Work out the finished part from the listing and answer in its coordinate system (mm). Round coordinates to 2 decimals unless told otherwise and drop trailing zeros. Loops run counter-clockwise (first coordinate to the right, second up) from the corner with the lowest first, then second, coordinate; pieces in that order, holes last.
from build123d import *

# Parameters (mm, degrees)
F0_W       = 106.68
F0_H       = 208.28
F1_DEPTH   = 2.54
F2_SIZE    = 52.07
F3_SIZE2   = 52.2153074575
F3_SIZE    = 101.6
F3_2_SIZE2 = 52.2153074575
F3_2_SIZE  = 101.6


with BuildPart() as f1:
    # F0 (on Top) → F1 (new body)
    with BuildSketch(Plane.XY):
        Rectangle(F0_W, F0_H)
    extrude(amount=F1_DEPTH)

    # F2
    f2_edges = [f1.edges().sort_by_distance(p)[0] for p in [
        (-53.34, -104.14, 1.27),
        (53.34, -104.14, 1.27),
    ]]
    chamfer(f2_edges, length=F2_SIZE)

    # F3
    f3_edges = [f1.edges().sort_by_distance(p)[0] for p in [
        (-53.34, 104.14, 1.27),
    ]]
    f3_side = f1.faces().sort_by_distance((-53.34, 26.035, 1.27))[0]
    chamfer(f3_edges, length=F3_SIZE, length2=F3_SIZE2, reference=f3_side)

    # F3#2
    f3_2_edges = [f1.edges().sort_by_distance(p)[0] for p in [
        (53.34, 104.14, 1.27),
    ]]
    f3_2_side = f1.faces().sort_by_distance((53.34, 26.035, 1.27))[0]
    chamfer(f3_2_edges, length=F3_2_SIZE, length2=F3_2_SIZE2, reference=f3_2_side)


solid = f1.part
Item 1: Section A-A, the plane z = 1.3 is taken. Give the vertices of the cut face in (x, y), plus the area to 3 significant figures.
Item 2: Section C-C, the plane x = -6 is taken. Give the vertices of the cut face in (y, z).
Item 3: Section B-B, the plane y = -67.5 is taken. Give the vertices of the cut face in (x, z), plus the area to 3 significant figures.
Item 4: Straight lines are drawn through the part: line 1 (Y direction, x = 7, z = 1.55); line 2 (X direction, y = -63, z = 0.35); line 3 (X direction, y = 87, z = 1.25). For each, find the intervals that lie inside material, in ascending order.
Item 5: Each of these flat-tipped pins is pushed along its axis until it touches: P1, Ø1, axis at y = 33, z = 2, coming from the +X side; P2, Ø1.5, axis at y = 77, z = 0.5, coming from the -X side. Where does it stop, or does it pass through?
Answer below:
1. outline: (-53.34, -52.07) - (-1.27, -104.14) - (1.27, -104.14) - (53.34, -52.07) - (53.34, 2.54) - (1.12, 104.14) - (-1.12, 104.14) - (-53.34, 2.54) - close
1. area: 14,200 mm2
2. outline: (-99.41, 0) - (94.65, 0) - (94.65, 2.54) - (-99.41, 2.54) - close
3. outline: (-37.91, 0) - (37.91, 0) - (37.91, 2.54) - (-37.91, 2.54) - close
3. area: 193 mm2
4. line 1: y = -98.41 to 92.71
4. line 2: x = -42.41 to 42.41
4. line 3: x = -9.93 to 9.93
5. P1: stops at x = 37.94
5. P2: stops at x = -15.46
